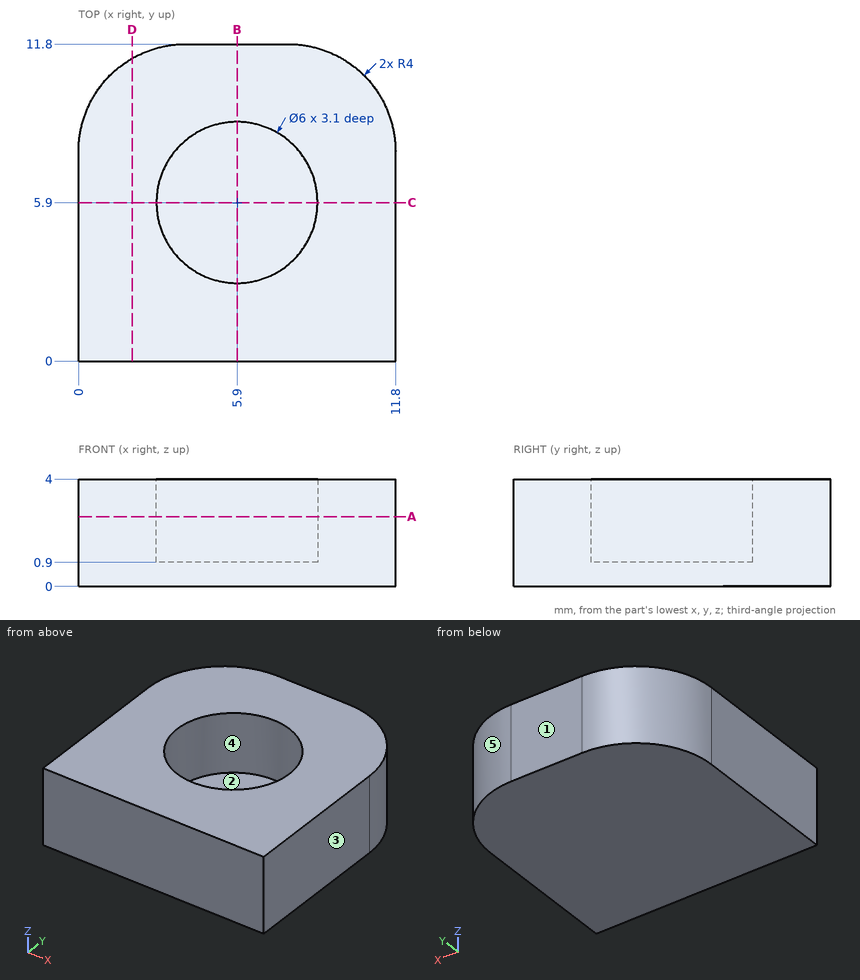
Study the drawing (mm; zero at the part's minimum x, y, z) and answer. A direction names the side the tool comes from. Round coordinates to 2 decimals unless told otherwise and drop trailing zeros. Loops run counter-clockwise (first coordinate to the right, second up) from the corner with the lowest first, then second, coordinate; pieces in that order, holes last.
Q1. Which of the six approach directions +Z, -Z, +X, -X, +Y, -Y give full straight-line access (tool end or side, diameter ignored) to the marked faces 1 and 2?
Q2. Section D-D, the plane x = 2 is taken. Determine the outline of the cut face in (y, z), then the cut area to 3 significant figures.
Q3. For a pull along Y with two mould halves and no side action, classify the marked faces 3, 4 and 5 as released by +Y, released by -Y, zero draft, split by the parting line, or undercut.
Q4. Given pin 1 Ø1.8 at (x, y) = (6.5, 4.5) entering from +Z, flat-ended and moving along its own axis, determine where the tip first touches the part or whether it passes through.
Q5. Find the intervals of material crossed by line 1 (Y direction, x = 5.9, z = 3.4); line 2 (Z direction, x = 8.25, y = 5.5); line 3 (X direction, y = 4, z = 1.75), in increasing order.
Q6. Section B-B, the plane x = 5.9 is taken. Determine the outline of the cut face in (y, z).
Q7. Section A-A, the plane z = 2.6 is taken. Determine the outline of the cut face in (x, y).
Completed:
1. face 1: +Z, -Z, +X, -X, +Y
1. face 2: +Z
2. outline: (0, 0) - (11.26, 0) - (11.26, 4) - (0, 4) - close
2. area: 45.1 mm2
3. face 3: zero draft
3. face 4: undercut
3. face 5: released by +Y
4. pin 1: stops at z = 0.9
5. line 1: y = 0 to 2.9, 8.9 to 11.8
5. line 2: z = 0 to 0.9
5. line 3: x = 0 to 3.58, 8.22 to 11.8
6. outline: (0, 0) - (11.8, 0) - (11.8, 4) - (8.9, 4) - (8.9, 0.9) - (2.9, 0.9) - (2.9, 4) - (0, 4) - close
7. outline: (0, 0) - (11.8, 0) - (11.8, 7.8) arc R4 ccw to (7.8, 11.8) - (4, 11.8) arc R4 ccw to (0, 7.8) - close; hole circle Ø6 at (5.9, 5.9)
